```python
from build123d import *

# Parameters (mm, degrees)
SKETCH1_W                       = 75
SKETCH1_H                       = 44
BOSS_EXTRUDE2_DEPTH             = 8
M4X0_7_TAPPED_HOLE2_D           = 3.3
M4X0_7_TAPPED_HOLE2_CSINK_D     = 4.05
M4X0_7_TAPPED_HOLE2_CSINK_ANGLE = 90


with BuildPart() as part:
    # Sketch1 → Boss-Extrude2 (new body)
    with BuildSketch(Plane(origin=(0, 0, 0), x_dir=(1, 0, 0), z_dir=(0, 1, 0))):
        with Locations((-16, 0)):
            Rectangle(SKETCH1_W, SKETCH1_H)
    extrude(amount=BOSS_EXTRUDE2_DEPTH)

    # M4x0.7 Tapped Hole2 (through all)
    with Locations(Plane.XY.offset(22)):
        with Locations((-46, 4), (14, 4)):
            CounterSinkHole(M4X0_7_TAPPED_HOLE2_D / 2, M4X0_7_TAPPED_HOLE2_CSINK_D / 2, counter_sink_angle=M4X0_7_TAPPED_HOLE2_CSINK_ANGLE)


solid = part.part
```
Geometry check sheet. Reference: the model listing, model coordinates, mm. Round coordinates to 2 decimals unless told otherwise and drop trailing zeros. Order: outer loops, then holes, each group sorted by start corner. A loop starts at its lowest first (then second) coordinate and runs counter-clockwise, first axis right, second up. Notation, with made-up numbers: (83.5, 64) -> (108.5, 64) arc R20 ccw to (108.5, 69) -> close; hole circle Ø10 at (7, 88.25). An arc over 180 degrees is marked (long way). Return JSON: item names as keys, results as strings. Group by question number.
Q1. Gauge pin test, flat end, axial feed: pin 1 (5 mm diameter, centred on x = -5.5, z = -7.5, fed in from -Y). Record the tip position at first contact, or that the pin passes through.
Q2. Release check for a two-part mould opening along X. For faces 1 (the cylindrical face through (12.476, 3.368, -0.493)), 2 (the flat face through (21.5, 4, 0)), 3 (the flat face through (-53.5, 4, 0)), 4 (the flat face through (-17, 8, 0)) record: released by +X, released by -X, zero draft, split by the parting line, or undercut.
Q3. Material ranges on probe 1 along X at (y, z) = (4, 3.5); probe 2 along Y at (x, z) = (-46, -4); probe 3 along X at (y, z) = (5.5, -3.5), recorded low to high. Write a range as from..to.
Q4. Section check C-C, the plane z = 6. Record the boundary of the cut face in (x, y).
Q5. Section check B-B, the plane x = 14. Record the boundary of the cut face in (y, z) (3 decimals), plus the area to 3 significant figures.
Q6. Section check A-A, the plane y = 4. Record the boundary of the cut face in (x, z) (3 decimals).
Numbers:
{
 "1": {"pin 1": "y = 0"},
 "2": {"face 1": "undercut", "face 2": "released by +X", "face 3": "released by -X", "face 4": "zero draft"},
 "3": {"probe 1": "-53.5..-47.65, -44.35..12.35, 15.65..21.5", "probe 2": "0..2.35, 5.65..8", "probe 3": "-53.5..-46.69, -45.31..13.31, 14.69..21.5"},
 "4": {"outline": "(-53.5, 0) -> (21.5, 0) -> (21.5, 8) -> (-53.5, 8) -> close; hole circle Ø3.3 at (-46, 4); hole circle Ø3.3 at (14, 4)"},
 "5": {"outline": "(0, -22) -> (2.35, -22) -> (2.35, 21.625) -> (1.975, 22) -> (0, 22) -> close; (5.65, -22) -> (8, -22) -> (8, 22) -> (6.025, 22) -> (5.65, 21.625) -> close", "area": "207 mm^2"},
 "6": {"outline": "(-53.5, -22) -> (-47.65, -22) -> (-47.65, 21.625) -> (-48.025, 22) -> (-53.5, 22) -> close; (-44.35, -22) -> (12.35, -22) -> (12.35, 21.625) -> (11.975, 22) -> (-43.975, 22) -> (-44.35, 21.625) -> close; (15.65, -22) -> (21.5, -22) -> (21.5, 22) -> (16.025, 22) -> (15.65, 21.625) -> close"}
}
